Input: dimensioned drawing with shaded views. Units: mm. Origin: part minimum x, y, z. Round coordinates to 2 decimals unless told otherwise and drop trailing zeros. Loops run counter-clockwise (first coordinate to the right, second up) from the corner with the lowest first, then second, coordinate; pieces in that order, holes last. Notation, with made-up numbers: (36, -33) - (55, -33) arc R21 cw to (55, -18) - close; hole circle Ø2 at (17.5, 4.25). An arc over 180 degrees is marked (long way). One line per question, with ' | ' between items. Start each with the question number.
Item 1: Section D-D, the plane y = 16.75. Return loops of the section in (x, z), plus the area to 3 significant figures.
Item 2: Section A-A, the plane y = 1.8. Return loops of the section in (x, z), plus the area to 3 significant figures.
Item 3: Section C-C, the plane z = 0.3. Return loops of the section in (x, y).
Item 4: First-contact query: pin 1 (1.5 mm diameter, centred on x = 8, y = 16.75, fed in from +Z); pin 2 (3 mm diameter, centred on x = 8, y = 16, fed in from +Z); pin 3 (3 mm diameter, centred on x = 8.5, y = 1.5, fed in from +Z). Flat tips, straight axial feed; report the tip coordinate or a pass-through.
Item 5: Section B-B, the plane x = 8. Return loops of the section in (y, z).
Item 6: Material intervals for line 1 along Y through (x, z) = (8, 0.7); line 2 along X through (y, z) = (16.75, 0.65); line 3 along X through (y, z) = (16.75, 1.5), sorted ascending.
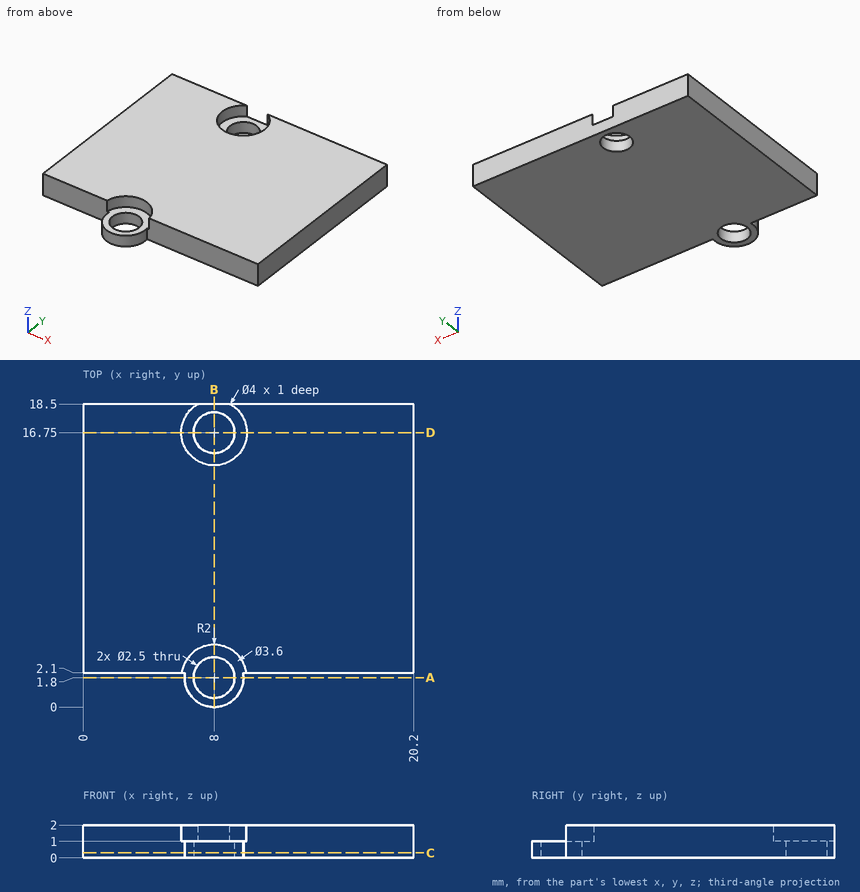
Return value:
1) outline: (0, 0) - (6.75, 0) - (6.75, 1) - (6, 1) - (6, 2) - (0, 2) - close; (9.25, 0) - (20.2, 0) - (20.2, 2) - (10, 2) - (10, 1) - (9.25, 1) - close | area: 33.9 mm2
2) outline: (6.2, 0) - (6.75, 0) - (6.75, 1) - (6.2, 1) - close; (9.25, 0) - (9.8, 0) - (9.8, 1) - (9.25, 1) - close | area: 1.10 mm2
3) outline: (0, 2.1) - (6.23, 2.1) arc R1.8 ccw (long way) to (9.77, 2.1) - (20.2, 2.1) - (20.2, 18.5) - (0, 18.5) - close; hole circle Ø2.5 at (8, 1.8); hole circle Ø2.5 at (8, 16.75)
4) pin 1: through | pin 2: z = 2 | pin 3: z = 1
5) outline: (0, 0) - (0.55, 0) - (0.55, 1) - (0, 1) - close; (3.05, 0) - (15.5, 0) - (15.5, 1) - (14.75, 1) - (14.75, 2) - (3.8, 2) - (3.8, 1) - (3.05, 1) - close; (18, 0) - (18.5, 0) - (18.5, 1) - (18, 1) - close
6) line 1: 0 to 0.55, 3.05 to 15.5, 18 to 18.5 | line 2: 0 to 6.75, 9.25 to 20.2 | line 3: 0 to 6, 10 to 20.2
